from build123d import *

# Parameters (mm, degrees)
SKETCH1_R                = 22.7203
BOSS_EXTRUDE2_DEPTH      = 4.7625
FILLET1_R                = 3.175
SKETCH2_W                = 14.732
SKETCH2_H                = 10.414
CUT_EXTRUDE2_DEPTH       = 12.7
CIRPATTERN1_COUNT        = 5
SKETCH4_R                = 1.143
CUT_EXTRUDE4_DEPTH       = 9.525
CIRPATTERN2_COUNT        = 5
SKETCH5_W                = 6.477
SKETCH5_H                = 6.477
CUT_EXTRUDE5_DEPTH       = 33.480350535
SKETCH6_R                = 2.286
CUT_EXTRUDE7_DEPTH       = 33.480350535
SKETCH7_R                = 4.445
CUT_EXTRUDE8_DEPTH       = 2.54
BOSS_EXTRUDE4_REACH      = 39.999
FILLET2_R                = 0.127
CIRPATTERN5_COUNT        = 5
FILLET2_OF_CIRPATTERN5_R = 0.127
FILLET3_R                = 1.016


with BuildPart() as part:
    # Sketch1 → Boss-Extrude2 (new body)
    with BuildSketch(Plane.XY):
        Circle(SKETCH1_R)
    extrude(amount=-BOSS_EXTRUDE2_DEPTH)

    # Fillet1
    fillet1_edges = [part.edges().sort_by_distance(p)[0] for p in [
        (-22.7203, 0, -4.7625),
    ]]
    fillet(fillet1_edges, radius=FILLET1_R)

    # Sketch2 → Cut-Extrude2 (cut)
    with BuildSketch(Plane.XY):
        with Locations((0, 18.7833)):
            Rectangle(SKETCH2_W, SKETCH2_H)
    cut_extrude2 = extrude(amount=-CUT_EXTRUDE2_DEPTH, mode=Mode.SUBTRACT)

    # CirPattern1: Cut-Extrude2 ×5 about axis
    cirpattern1_axis = Axis((0, 0, 0), (0, 0, 1))
    for i in range(1, CIRPATTERN1_COUNT):
        add(cut_extrude2.rotate(cirpattern1_axis, i * 360 / CIRPATTERN1_COUNT), mode=Mode.SUBTRACT)

    # Sketch4 → Cut-Extrude4 (cut, symmetric)
    with BuildSketch(Plane(origin=(0, 0, 0), x_dir=(0, 0, -1), z_dir=(1, 0, 0))):
        with Locations((0, 19.4183)):
            Circle(SKETCH4_R)
    cut_extrude4 = extrude(amount=CUT_EXTRUDE4_DEPTH, both=True, mode=Mode.SUBTRACT)

    # CirPattern2: Cut-Extrude4 ×5 about axis
    cirpattern2_axis = Axis((0, 0, 0), (0, 0, 1))
    for i in range(1, CIRPATTERN2_COUNT):
        add(cut_extrude4.rotate(cirpattern2_axis, i * 360 / CIRPATTERN2_COUNT), mode=Mode.SUBTRACT)

    # Sketch5 → Cut-Extrude5 (cut, through all)
    with BuildSketch(Plane.XY):
        Rectangle(SKETCH5_W, SKETCH5_H)
    extrude(amount=-CUT_EXTRUDE5_DEPTH, mode=Mode.SUBTRACT)

    # Sketch6 → Cut-Extrude7 (cut, through all)
    with BuildSketch(Plane(origin=(0, 0, -4.7625), x_dir=(-1, 0, 0), z_dir=(0, 0, -1))):
        with Locations((0, 8.89)):
            Circle(SKETCH6_R)
        with Locations((8.89, 0)):
            Circle(SKETCH6_R)
        with Locations((0, -8.89)):
            Circle(SKETCH6_R)
        with Locations((-8.89, 0)):
            Circle(SKETCH6_R)
    extrude(amount=-CUT_EXTRUDE7_DEPTH, mode=Mode.SUBTRACT)

    # Sketch7 → Cut-Extrude8 (cut)
    with BuildSketch(Plane(origin=(0, 0, -4.7625), x_dir=(-1, 0, 0), z_dir=(0, 0, -1))):
        with Locations((-8.89, 0)):
            Circle(SKETCH7_R)
        with Locations((8.89, 0)):
            Circle(SKETCH7_R)
        with Locations((0, -8.89)):
            Circle(SKETCH7_R)
        with Locations((0, 8.89)):
            Circle(SKETCH7_R)
    extrude(amount=-CUT_EXTRUDE8_DEPTH, mode=Mode.SUBTRACT)

    # Sketch10 → Boss-Extrude4 (add, up to next)
    with BuildSketch(Plane.ZY.offset(-7.366), mode=Mode.PRIVATE) as boss_extrude4_sk1:
        with BuildLine():
            Line((-4.7625, 13.5763), (0, 13.5763))
            Line((0, 13.5763), (0, 13.7033))
            ThreePointArc((0, 13.7033), (-2.7025038, 14.38265722), (-4.7625, 16.259214887))
            Line((-4.7625, 16.259214887), (-4.7625, 13.5763))
        make_face()
    boss_extrude4_tool1 = extrude(boss_extrude4_sk1.sketch, amount=BOSS_EXTRUDE4_REACH, mode=Mode.PRIVATE) - part.part
    boss_extrude4 = boss_extrude4_tool1.solids().sort_by_distance((7.366, 14.314807, -3.452063))[0]
    add(boss_extrude4)

    # Fillet2
    fillet2_edges = [part.edges().sort_by_distance(p)[0] for p in [
        (0, 16.259214887, -4.7625),
    ]]
    fillet(fillet2_edges, radius=FILLET2_R)

    # CirPattern5: Boss-Extrude4 ×5 about axis
    cirpattern5_axis = Axis((0, 0, 0), (0, 0, 1))
    for i in range(1, CIRPATTERN5_COUNT):
        add(boss_extrude4.rotate(cirpattern5_axis, i * 360 / CIRPATTERN5_COUNT))

    # Fillet2 of CirPattern5
    fillet2_of_cirpattern5_edges = [part.edges().sort_by_distance(p)[0] for p in [
        (-15.463432268, 5.024373715, -4.7625),
        (-9.556926725, -13.153981159, -4.7625),
        (9.556926725, -13.153981159, -4.7625),
        (15.463432268, 5.024373715, -4.7625),
    ]]
    fillet(fillet2_of_cirpattern5_edges, radius=FILLET2_OF_CIRPATTERN5_R)

    # Fillet3
    fillet3_edges = [part.edges().sort_by_distance(p)[0] for p in [
        (3.2385, 3.2385, -2.38125),
        (3.2385, -3.2385, -2.38125),
        (-3.2385, -3.2385, -2.38125),
        (-3.2385, 3.2385, -2.38125),
    ]]
    fillet(fillet3_edges, radius=FILLET3_R)


solid = part.part
The listing builds one solid part. Answer for the finished solid, in the listing's coordinates (mm). A direction names the side the tool comes from. Give positions to 0.01 mm unless a question says otherwise; leave off trailing zeros.
Item 1: A tool of negligible diameter and unlimited length cuts with its end or side. For faces 4 (the flat face through (-11, -2, -2.222)), 5 (the flat face through (-18.961, -1.584, -2.348)), 6 (the flat face through (3.238, 0, -2)), from which of +Z, -Z, +X, -X, +Y, -Y can it reach the whole face along a straight path? Write none if from no direction.
Derived:
face 4: -Z
face 5: +Z
face 6: +Z, -Z
Item 2: Find the intervals of material crossed by line 1 along Y through (x, z) = (8.89, -0.5); line 2 along X through (y, z) = (-7, -0.65); line 3 along Y through (x, z) = (-3, -1.5), in increasing order.
Derived:
line 1: y = -10.51 to -2.29, 2.29 to 18.39, 20.45 to 20.91
line 2: x = -21.62 to -14.19, -13.74 to -1.29, 1.29 to 13.74, 14.19 to 21.62
line 3: y = -22.52 to -16.66, -15.01 to -2.88, 2.88 to 13.9
Item 3: Determine the mould class of faces 1 (the cylindrical face through (21.58, -7.11, -0.78)), 2 (the flat face through (7.366, 18, -2)), 3 (the flat face through (-4.35, -18.52, -2.35)) for opening direction X: +X half, -X half, draft (parallel to the pull), parting line (faces both ways), or undercut.
Derived:
face 1: +X half
face 2: undercut
face 3: -X half
Item 4: A cutting plane is placed at A-A (x = 0). Give the number of separate pieces and of enclosed holes in the cut face, then the cut area to 3 significant figures.
Derived:
separate pieces: 4
enclosed holes: 0
area: 78.6 mm2
Item 5: Each of these flat-tipped pins is pushed along its axis until it touches: pin 1 Ø2 at (y, z) = (13, -3) entering from +X; pin 2 Ø4.5 at (x, y) = (-9, 1.5) entering from -Z; pin 3 Ø2 at (x, z) = (-8, -1.5) entering from -Y. Where does it stop, or does it pass through?
Derived:
pin 1: stops at x = 18.1
pin 2: stops at z = -2.22
pin 3: stops at y = -12.2
